Design review of the part built by this model. Coordinates are the model's own, in mm. A direction names the side the tool comes from. Round coordinates to 2 decimals unless told otherwise and drop trailing zeros. Order: outer loops, then holes, each group sorted by start corner. A loop starts at its lowest first (then second) coordinate and runs counter-clockwise, first axis right, second up.
from build123d import *

# Parameters (mm, degrees)
SZKIC1_W                        = 27
SZKIC1_H                        = 25
ZAOKR_GLENIE1_R                 = 4
SZKIC4_R                        = 3
WYTNIJ_WYCI_GNI_CIE3_DEPTH      = 24.0000001
WYTNIJ_WYCI_GNI_CIE3_DEPTH_BACK = 3
WYTNIJ_WYCI_GNI_CIE2_DEPTH      = 24.0000001
SZKIC5_OUTSIDE_W                = 72.072
SZKIC5_OUTSIDE_H                = 72.072
WYTNIJ_WYCI_GNI_CIE4_DEPTH      = 26.0000001
SZKIC8_W                        = 7.75
SZKIC8_H                        = 9.576606241
SZKIC10_R                       = 3.5
WYTNIJ_WYCI_GNI_CIE5_DEPTH      = 56.423393859


with BuildPart() as part:
    # Szkic1 → Obrót1 (revolve)
    with BuildSketch(Plane.XY):
        with Locations((13.5, 12.5)):
            Rectangle(SZKIC1_W, SZKIC1_H)
    revolve(axis=Axis((0, 0, 0), (0, 1, 0)))

    # Szkic2 → Wycięcie-obrót1 (revolve, cut)
    with BuildSketch(Plane.XY):
        Polygon((27, 25), (27, 2), (7.75, 13.113992682), (7.75, 25), align=None)
    revolve(axis=Axis((0, 0, 0), (0, 1, 0)), mode=Mode.SUBTRACT)

    # Zaokrąglenie1
    zaokr_glenie1_edges = [part.edges().sort_by_distance(p)[0] for p in [
        (-7.75, 13.113992682, 0),
    ]]
    fillet(zaokr_glenie1_edges, radius=ZAOKR_GLENIE1_R)

    # Szkic4 → Wytnij-wyciągnięcie3 (cut, two sides)
    with BuildSketch(Plane(origin=(0, 2, 0), x_dir=(1, 0, 0), z_dir=(0, 1, 0))) as wytnij_wyci_gni_cie3_sk:
        with Locations((-20, 0)):
            Circle(SZKIC4_R)
        with Locations((20, 0)):
            Circle(SZKIC4_R)
    extrude(amount=WYTNIJ_WYCI_GNI_CIE3_DEPTH, mode=Mode.SUBTRACT)
    extrude(wytnij_wyci_gni_cie3_sk.sketch, amount=-WYTNIJ_WYCI_GNI_CIE3_DEPTH_BACK, mode=Mode.SUBTRACT)

    # Szkic3 → Wytnij-wyciągnięcie2 (cut, through all)
    with BuildSketch(Plane(origin=(0, 2, 0), x_dir=(1, 0, 0), z_dir=(0, 1, 0))):
        with BuildLine():
            Line((-17.5, 5), (-26.532998323, 5))
            ThreePointArc((-26.532998323, 5), (-27, 0), (-26.532998323, -5))
            Line((-26.532998323, -5), (-17.5, -5))
            ThreePointArc((-17.5, -5), (-12.5, 0), (-17.5, 5))
        make_face()
        with BuildLine():
            Line((17.5, 5), (26.532998323, 5))
            ThreePointArc((26.532998323, 5), (27, 0), (26.532998323, -5))
            Line((26.532998323, -5), (17.5, -5))
            ThreePointArc((17.5, -5), (12.5, 0), (17.5, 5))
        make_face()
    extrude(amount=WYTNIJ_WYCI_GNI_CIE2_DEPTH, mode=Mode.SUBTRACT)

    # Szkic5 outside → Wytnij-wyciągnięcie4 (cut, through all)
    with BuildSketch(Plane.XZ):
        Rectangle(SZKIC5_OUTSIDE_W, SZKIC5_OUTSIDE_H)
        with BuildLine():
            Line((-20.2625, 6.995076393), (-0.290625, 7.744548864))
            ThreePointArc((-0.290625, 7.744548864), (0, 7.75), (0.290625, 7.744548864))
            Line((0.290625, 7.744548864), (20.2625, 6.995076393))
            ThreePointArc((20.2625, 6.995076393), (27, 0), (20.2625, -6.995076393))
            Line((20.2625, -6.995076393), (0.290625, -7.744548864))
            ThreePointArc((0.290625, -7.744548864), (0, -7.75), (-0.290625, -7.744548864))
            Line((-0.290625, -7.744548864), (-20.2625, -6.995076393))
            ThreePointArc((-20.2625, -6.995076393), (-27, 0), (-20.2625, 6.995076393))
        make_face(mode=Mode.SUBTRACT)
    extrude(amount=-WYTNIJ_WYCI_GNI_CIE4_DEPTH, mode=Mode.SUBTRACT)

    # Szkic8 → Wycięcie-obrót2 (revolve, cut)
    with BuildSketch(Plane.XY):
        with Locations((3.875, 20.211696879)):
            Rectangle(SZKIC8_W, SZKIC8_H)
    revolve(axis=Axis((0, 25, 0), (0, -1, 0)), mode=Mode.SUBTRACT)

    # Szkic9 → Obrót2 (revolve)
    with BuildSketch(Plane.XY):
        Polygon((0, 15.423393759), (0, 55.423393759), (5.35, 55.423393759), (6.35, 54.423393759), (6.35, 52.423393759), (6.3, 52.423393759), (6.3, 15.423393759), align=None)
    revolve(axis=Axis((0, 15.423393759, 0), (0, 1, 0)))

    # Szkic10 → Wytnij-wyciągnięcie5 (cut, through all)
    with BuildSketch(Plane(origin=(0, 55.423393759, 0), x_dir=(1, 0, 0), z_dir=(0, 1, 0))):
        Circle(SZKIC10_R)
    extrude(amount=-WYTNIJ_WYCI_GNI_CIE5_DEPTH, mode=Mode.SUBTRACT)


solid = part.part
1) To check wall thickness, follow line 1 along X through (y, z) = (1.55, 0); line 2 along Z through (x, y) = (0, 25); line 3 along Z through (x, y) = (20, 1.25). State the ranges of each line that lie inside material, in increasing order.
Results:
line 1: x = -27 to -23, -17 to -3.5, 3.5 to 17, 23 to 27
line 2: z = -6.3 to -3.5, 3.5 to 6.3
line 3: z = -7 to -3, 3 to 7
2) Take a section at B-B on z = 1. State how many separate pieces and enclosed holes the cut face has, plus the area to 3 significant figures.
Results:
separate pieces: 4
enclosed holes: 0
area: 514 mm2
3) The part is to be moulded in two halves that separate along X. For faces 1 (the face through (27, 1, 0)), 2 (the face through (17, 1, 0)), 3 (the face through (-20, 4, 5)), 4 (the face through (-1.38, 53.41, 6.2)), say which applies: released by +X, released by -X, zero draft, split by the parting line, or undercut.
Results:
face 1: released by +X
face 2: undercut
face 3: zero draft
face 4: split by the parting line
4) For faces 5 (the face through (-8.197, 5.887, 7.448)), 6 (the face through (-12.5, 5.2, 0.1)), 7 (the face through (20, 4, 5)), list the 3-axis set-ups (+Z, -Z, +X, -X, +Y, -Y) from which the entire face can be reached by the end or side of a thin tool; tool diameter is ignored.
Results:
face 5: +Z, -X, +Y, -Y
face 6: -X, +Y
face 7: +X, +Y
5) Take a section at A-A on y = 44. Give the boundary of the cut face in (x, z).
Results:
outline: circle Ø12.6 at (0, 0); hole circle Ø7 at (0, 0)
6) Clearance check with flat-ended pins moving along their axes: P1, Ø4, axis at x = -20.5, y = 4.5, coming from the -Z side; P2, Ø4, axis at x = 22.5, y = 3.5, coming from the +Z side; P3, Ø5, axis at x = -22.5, z = 1.5, coming from the +Y side; P4, Ø5.5, axis at x = -20, z = 0, coming from the +Y side. State where each tip first meets the part, or that it passes through.
Results:
P1: stops at z = -7.06
P2: stops at z = 6.98
P3: stops at y = 2
P4: passes through
